Can you work these out from the model? Positions are in its coordinate system, mm. Face numbers are marked on the shaded views. A direction names the side the tool comes from. Round coordinates to 2 decimals unless told otherwise and drop trailing zeros. Order: outer loops, then holes, each group sorted by start corner. A loop starts at its lowest first (then second) coordinate and runs counter-clockwise, first axis right, second up. Notation, with made-up numbers: M 59.5,57 L 111.5,57 A26 cw 111.5,76 Z; hole C 50.25,28.25 d4. An arc over 180 degrees is marked long. One line per question, with ' | ' between items.
```python
from build123d import *

# Parameters (mm, degrees)
SKETCH1_R           = 41
SKETCH1_R_2         = 3
BOSS_EXTRUDE1_DEPTH = 40
SKETCH2_R           = 7.9
BOSS_EXTRUDE2_DEPTH = 20
FILLET1_R           = 10
FILLET2_R           = 0.5
SKETCH3_R           = 57.838297584
SKETCH3_R_2         = 26
CUT_EXTRUDE1_DEPTH  = 35
FILLET3_R           = 4
FILLET4_R           = 0.5
SKETCH5_R           = 25
CUT_EXTRUDE2_DEPTH  = 35
CHAMFER1_SIZE       = 3


with BuildPart() as part:
    # Sketch1 → Boss-Extrude1 (new body)
    with BuildSketch(Plane(origin=(0, 0, 0), x_dir=(0, 0, -1), z_dir=(1, 0, 0))):
        Circle(SKETCH1_R)
        with Locations((0, 30)):
            Circle(SKETCH1_R_2, mode=Mode.SUBTRACT)
        with Locations((25.980762114, 15)):
            Circle(SKETCH1_R_2, mode=Mode.SUBTRACT)
        with Locations((25.980762114, -15)):
            Circle(SKETCH1_R_2, mode=Mode.SUBTRACT)
        with Locations((0, -30)):
            Circle(SKETCH1_R_2, mode=Mode.SUBTRACT)
        with Locations((-25.980762114, -15)):
            Circle(SKETCH1_R_2, mode=Mode.SUBTRACT)
        with Locations((-25.980762114, 15)):
            Circle(SKETCH1_R_2, mode=Mode.SUBTRACT)
    extrude(amount=BOSS_EXTRUDE1_DEPTH)

    # Sketch2 → Boss-Extrude2 (add)
    with BuildSketch(Plane.ZY):
        with Locations(Location((0, 0, 0), (0, 0, 180))):
            Circle(SKETCH2_R)
    extrude(amount=BOSS_EXTRUDE2_DEPTH)

    # Fillet1
    fillet1_edges = [part.edges().sort_by_distance(p)[0] for p in [
        (0, 0, 7.9),
    ]]
    fillet(fillet1_edges, radius=FILLET1_R)

    # Fillet2
    fillet2_edges = [part.edges().sort_by_distance(p)[0] for p in [
        (0, 0, 41),
        (40, 0, 41),
    ]]
    fillet(fillet2_edges, radius=FILLET2_R)

    # Sketch3 → Cut-Extrude1 (cut)
    with BuildSketch(Plane(origin=(0, 0, 0), x_dir=(0, 0, -1), z_dir=(1, 0, 0))):
        Circle(SKETCH3_R)
        Circle(SKETCH3_R_2, mode=Mode.SUBTRACT)
    extrude(amount=CUT_EXTRUDE1_DEPTH, mode=Mode.SUBTRACT)

    # Fillet3
    # the kernel refuses this fillet: 4 mm, written as the material it adds along each edge
    with BuildSketch(Plane(origin=(35, 0, 0), x_dir=(0, 0, -1), z_dir=(0, -1, 0))) as fillet3_piece_1_section:
        with BuildLine():
            CenterArc((26 + FILLET3_R, -FILLET3_R), FILLET3_R, 90, 90)
            Line((26 + FILLET3_R, 0), (26, 0))
            Line((26, 0), (26, -FILLET3_R))
        make_face()
    fillet3_piece_1 = revolve(axis=Axis((35, 0, 0), (1, 0, 0)), mode=Mode.PRIVATE)
    fillet3_piece_1 = fillet3_piece_1 - Plane(origin=(33.889931495, -15, 25.980762114), x_dir=(0, 0, -1), z_dir=(-1, 0, 0)) * Cylinder(3, 120, mode=Mode.PRIVATE)
    fillet3_piece_1 = fillet3_piece_1 - Plane(origin=(33.889931495, -30, 0), x_dir=(0, 0, -1), z_dir=(-1, 0, 0)) * Cylinder(3, 120, mode=Mode.PRIVATE)
    fillet3_piece_1 = fillet3_piece_1 - Plane(origin=(33.889931495, -15, -25.980762114), x_dir=(0, 0, -1), z_dir=(-1, 0, 0)) * Cylinder(3, 120, mode=Mode.PRIVATE)
    fillet3_piece_1 = fillet3_piece_1 - Plane(origin=(33.889931495, 15, 25.980762114), x_dir=(0, 0, -1), z_dir=(-1, 0, 0)) * Cylinder(3, 120, mode=Mode.PRIVATE)
    fillet3_piece_1 = fillet3_piece_1 - Plane(origin=(33.889931495, 15, -25.980762114), x_dir=(0, 0, -1), z_dir=(-1, 0, 0)) * Cylinder(3, 120, mode=Mode.PRIVATE)
    fillet3_piece_1 = fillet3_piece_1 - Plane(origin=(33.889931495, 30, 0), x_dir=(0, 0, -1), z_dir=(-1, 0, 0)) * Cylinder(3, 120, mode=Mode.PRIVATE)
    add(fillet3_piece_1)

    # Fillet4
    fillet4_edges = [part.edges().sort_by_distance(p)[0] for p in [
        (0, 0, 26),
    ]]
    fillet(fillet4_edges, radius=FILLET4_R)

    # Sketch5 → Cut-Extrude2 (cut)
    with BuildSketch(Plane(origin=(40, 0, 0), x_dir=(0, 0, -1), z_dir=(1, 0, 0))):
        Circle(SKETCH5_R)
    extrude(amount=-CUT_EXTRUDE2_DEPTH, mode=Mode.SUBTRACT)

    # Chamfer1
    # the kernel refuses this chamfer: 3 mm, written as the material it takes off along each edge
    with BuildSketch(Plane(origin=(40, 0, 0), x_dir=(0, 0, -1), z_dir=(0, -1, 0))) as chamfer1_piece_1:
        Polygon((25 + CHAMFER1_SIZE, 0), (25, -CHAMFER1_SIZE), (25, 0), align=None)
    revolve(axis=Axis((40, 0, 0), (1, 0, 0)), mode=Mode.SUBTRACT)


solid = part.part
```
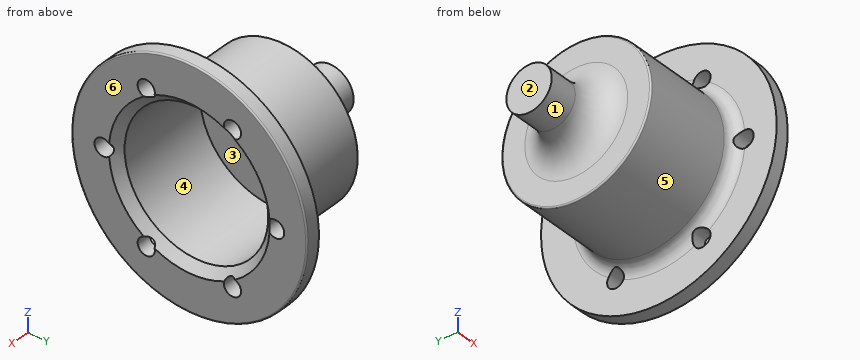
(1) On a 3-axis mill with a long thin cutter (end or side, diameter ignored), from which of +Z, -Z, +X, -X, +Y, -Y can I reach the whole of each face in a straight line? I mean the marked faces 4, 5 and 6. Say none if no direction works.
Final values:
face 4: +X | face 5: -X | face 6: +Z, -Z, +X, +Y, -Y
(2) If we section it at B-B on y = 0: Please give me the cut outline in (x, z).
Final values:
outline: M -20,-7.9 L -10,-7.9 A10 cw 0,-17.9 L 0,-25.5 A0.5 ccw 0.5,-26 L 31,-26 A4 cw 35,-30 L 35,-41 L 39.5,-41 A0.5 ccw 40,-40.5 L 40,-28 L 37,-25 L 5,-25 L 5,25 L 37,25 L 40,28 L 40,40.5 A0.5 ccw 39.5,41 L 35,41 L 35,30 A4 cw 31,26 L 0.5,26 A0.5 ccw 0,25.5 L 0,17.9 A10 cw -10,7.9 L -20,7.9 Z
(3) If we section it at D-D on x = -14.5: Please give me the cut outline in (y, z), plus the area to 3 significant figures.
Final values:
outline: C 0,0 d15.8 | area: 196 mm^2
(4) If we section it at C-C on x = 17: Please give me the cut outline in (y, z), plus the area to 3 significant figures.
Final values:
outline: C 0,0 d52; hole C 0,0 d50 | area: 160 mm^2
(5) Thinking about a two-plate mould opening in Y: for the marked faces 1, 2 and 3, which applies, released by +Y, released by -Y, zero draft, split by the parting line, or undercut?
Final values:
face 1: split by the parting line | face 2: zero draft | face 3: undercut
(6) Will these pins go through, and if not, where does the flat tip stop? pin 1 Ø6 at (x, y) = (16.5, 26) entering from +Z; pin 2 Ø1.5 at (y, z) = (-12.5, 27) entering from -X; pin 3 Ø6 at (x, y) = (27, -1.5) entering from -Z; pin 4 Ø9.5 at (y, z) = (-15, 25.98) entering from +X.
Final values:
pin 1: z = 12.12 | pin 2: x = 34.88 | pin 3: z = -26 | pin 4: x = 40
(7) Please list where these lines run through material, in increasing order: probe 1 along Z at (x, y) = (38, -30); probe 2 along X at (y, z) = (-16, -33); probe 3 along Y at (x, z) = (15, 0). Write a range as [from, to].
Final values:
probe 1: [-27.95, -3], [3, 27.95] | probe 2: [35, 40] | probe 3: [-26, -25], [25, 26]
(8) If we section it at A-A on z = 0: State how many separate pieces and enclosed holes the cut face has, plus the area to 3 significant figures.
Final values:
separate pieces: 3 | enclosed holes: 0 | area: 775 mm^2
